Verification items for the finished model (mm, model axes). A direction names the side the tool comes from. Give positions to 0.01 mm unless a question says otherwise; leave off trailing zeros. Write each loop counter-clockwise with the first axis right and the second up, starting at its lowest first coordinate (ties: lowest second). Pieces come first, ordered by that corner, then holes. Notation, with made-up numbers: (87, 69.25) -> (108, 69.25) arc R24 cw to (108, 84.25) -> close; hole circle Ø6 at (-29, 32). An arc over 180 degrees is marked (long way). Write item = value, one per line.
from build123d import *

# Parameters (mm, degrees)
SKETCH_1_R          = 60
SKETCH_1_R_2        = 37.5
EXTRUDE_1_DEPTH     = 13
SKETCH_4_R          = 60
SKETCH_4_R_2        = 2
SKETCH_4_W          = 40
SKETCH_4_H          = 20
EXTRUDE_2_DEPTH     = 1
SKETCH_5_R          = 3.5
EXTRUDE_3_DEPTH     = 56
SKETCH_6_R          = 2
CUT_EXTRUDE_1_DEPTH = 5
SKETCH_7_R          = 45
CUT_EXTRUDE_2_DEPTH = 2


with BuildPart() as part:
    # Sketch 1 → Extrude 1 (new body)
    with BuildSketch(Plane.XY):
        with Locations(Location((0, 0, 0), (0, 0, 180))):
            Circle(SKETCH_1_R)
        with Locations(Location((0, 0, 0), (0, 0, 180))):
            Circle(SKETCH_1_R_2, mode=Mode.SUBTRACT)
    extrude(amount=EXTRUDE_1_DEPTH)



with BuildPart() as body_2:
    # Sketch 4 → Extrude 2 (new body)
    with BuildSketch(Plane.XY.offset(28)):
        with Locations(Location((0, 0, 0), (0, 0, 180))):
            Circle(SKETCH_4_R)
        with Locations((-15, 5)):
            Circle(SKETCH_4_R_2, mode=Mode.SUBTRACT)
        with Locations((35, 5)):
            Circle(SKETCH_4_R_2, mode=Mode.SUBTRACT)
        with Locations((35, -5)):
            Circle(SKETCH_4_R_2, mode=Mode.SUBTRACT)
        with Locations((-15, -5)):
            Circle(SKETCH_4_R_2, mode=Mode.SUBTRACT)
        with Locations((10, 0)):
            Rectangle(SKETCH_4_W, SKETCH_4_H, mode=Mode.SUBTRACT)
    extrude(amount=EXTRUDE_2_DEPTH)


with BuildPart() as part_1:
    add(part.part)

    add(body_2.part)  # Extrude 3 merges body 2
    # Sketch 5 → Extrude 3 (add)
    with BuildSketch(Plane.XY.offset(13)):
        with Locations((50, 0)):
            Circle(SKETCH_5_R)
        with Locations((0, -50)):
            Circle(SKETCH_5_R)
        with Locations((-50, 0)):
            Circle(SKETCH_5_R)
        with Locations((0, 50)):
            Circle(SKETCH_5_R)
    extrude(amount=EXTRUDE_3_DEPTH)

    # Sketch 6 → Cut-Extrude 1 (cut)
    with BuildSketch(Plane.XY.offset(69)):
        with Locations((50, 0)):
            Circle(SKETCH_6_R)
        with Locations((0, 50)):
            Circle(SKETCH_6_R)
        with Locations((-50, 0)):
            Circle(SKETCH_6_R)
        with Locations((0, -50)):
            Circle(SKETCH_6_R)
    extrude(amount=-CUT_EXTRUDE_1_DEPTH, mode=Mode.SUBTRACT)

    # Sketch 7 → Cut-Extrude 2 (cut)
    with BuildSketch(Plane(origin=(0, 0, 0), x_dir=(-1, 0, 0), z_dir=(0, 0, -1))):
        Circle(SKETCH_7_R)
    extrude(amount=-CUT_EXTRUDE_2_DEPTH, mode=Mode.SUBTRACT)


solid = part_1.part
Item 1: Go/stop test with flat-tipped pins: P1, Ø4.5, axis at x = -15, y = -5, coming from the +Z side; P2, Ø1.5, axis at x = -21, z = 12, coming from the +Y side; P3, Ø2, axis at x = 15.5, y = -18.5, coming from the -Z side. Record where each tip stops, or that it passes through.
Response values:
P1 = 29
P2 = 56.48
P3 = 28
Item 2: Mould release check, pull along Y, two halves, no side actions. Record for faces 1 (the cylindrical face through (-32.26, -50.59, 28.49)), 2 (the flat face through (-9, -45, 0)), 3 (the cylindrical face through (0.923, 48.226, 66.535)): +Y half, -Y half, draft (parallel to the pull), parting line (faces both ways), or undercut.
Response values:
face_1 = parting line
face_2 = draft
face_3 = undercut
Item 3: Sectioned sample at A-A on y = -29. Record the cut outline in (x, z).
Response values:
outline = (-52.53, 0) -> (-34.41, 0) -> (-34.41, 2) -> (-23.77, 2) -> (-23.77, 13) -> (-52.53, 13) -> close; (-52.53, 28) -> (52.53, 28) -> (52.53, 29) -> (-52.53, 29) -> close; (23.77, 2) -> (34.41, 2) -> (34.41, 0) -> (52.53, 0) -> (52.53, 13) -> (23.77, 13) -> close
Item 4: Sectioned sample at B-B on z = 62. Record the cut outline in (x, y), then the cut area to 3 significant figures.
Response values:
outline = circle Ø7 at (-50, 0); circle Ø7 at (0, -50); circle Ø7 at (0, 50); circle Ø7 at (50, 0)
area = 154 mm^2
Item 5: Sectioned sample at D-D on y = 5. Record the cut outline in (x, z), then the cut area to 3 significant figures.
Response values:
outline = (-59.79, 0) -> (-44.72, 0) -> (-44.72, 2) -> (-37.17, 2) -> (-37.17, 13) -> (-59.79, 13) -> close; (-59.79, 28) -> (-17, 28) -> (-17, 29) -> (-59.79, 29) -> close; (-13, 28) -> (-10, 28) -> (-10, 29) -> (-13, 29) -> close; (30, 28) -> (33, 28) -> (33, 29) -> (30, 29) -> close; (37, 28) -> (59.79, 28) -> (59.79, 29) -> (37, 29) -> close; (37.17, 2) -> (44.72, 2) -> (44.72, 0) -> (59.79, 0) -> (59.79, 13) -> (37.17, 13) -> close
area = 630 mm^2
Item 6: Set-up check for faces 4 (the cylindrical face through (-17.3, 33.27, 7.42)), 5 (the cylindrical face through (-16.6, -6.2, 28.5)), 6 (the cylindrical face through (-0.46, -46.53, 48.72)): record each of +Z, -Z, +X, -X, +Y, -Y from which the full face is reachable in a straight line by a thin tool's end or side.
Response values:
face_4 = -Z
face_5 = +Z, -Z
face_6 = +Z
Item 7: Material ranges on line 1 (Y direction, x = 0, z = 67.6); line 2 (Z direction, x = -47, y = 16); line 3 (Y direction, x = -50, z = 67), recorded low to high.
Response values:
line_1 = -53.5 to -52, -48 to -46.5, 46.5 to 48, 52 to 53.5
line_2 = 0 to 13, 28 to 29
line_3 = -3.5 to -2, 2 to 3.5
Item 8: Sectioned sample at C-C on x = 23. Record the cut outline in (y, z), then the cut area to 3 significant figures.
Response values:
outline = (-55.42, 0) -> (-38.68, 0) -> (-38.68, 2) -> (-29.62, 2) -> (-29.62, 13) -> (-55.42, 13) -> close; (-55.42, 28) -> (-10, 28) -> (-10, 29) -> (-55.42, 29) -> close; (10, 28) -> (55.42, 28) -> (55.42, 29) -> (10, 29) -> close; (29.62, 2) -> (38.68, 2) -> (38.68, 0) -> (55.42, 0) -> (55.42, 13) -> (29.62, 13) -> close
area = 725 mm^2
